```python
from build123d import *

# Parameters (mm, degrees)
SKETCH1_R           = 8
SKETCH1_R_2         = 1.5
SKETCH1_R_3         = 2
SKETCH1_W           = 10
SKETCH1_H           = 10
BOSS_EXTRUDE2_DEPTH = 8


with BuildPart() as part:
    # Sketch1 → Boss-Extrude2 (new body)
    with BuildSketch(Plane.XY):
        with BuildLine():
            Line((18.5, -45), (-18.5, -45))
            ThreePointArc((-18.5, -45), (-21.328427125, -43.828427125), (-22.5, -41))
            Line((-22.5, -41), (-22.5, 41))
            ThreePointArc((-22.5, 41), (-21.328427125, 43.828427125), (-18.5, 45))
            Line((-18.5, 45), (18.5, 45))
            ThreePointArc((18.5, 45), (21.328427125, 43.828427125), (22.5, 41))
            Line((22.5, 41), (22.5, -41))
            ThreePointArc((22.5, -41), (21.328427125, -43.828427125), (18.5, -45))
        make_face()
        Circle(SKETCH1_R, mode=Mode.SUBTRACT)
        with Locations((-11, 0)):
            Circle(SKETCH1_R_2, mode=Mode.SUBTRACT)
        with Locations((-5.5, 9.526279442)):
            Circle(SKETCH1_R_2, mode=Mode.SUBTRACT)
        with Locations((5.5, 9.526279442)):
            Circle(SKETCH1_R_2, mode=Mode.SUBTRACT)
        with Locations((11, 0)):
            Circle(SKETCH1_R_2, mode=Mode.SUBTRACT)
        with Locations((5.5, -9.526279442)):
            Circle(SKETCH1_R_2, mode=Mode.SUBTRACT)
        with Locations((-5.5, -9.526279442)):
            Circle(SKETCH1_R_2, mode=Mode.SUBTRACT)
        with Locations((0, -34.5)):
            Circle(SKETCH1_R_3, mode=Mode.SUBTRACT)
        with Locations((0, 34.5)):
            Circle(SKETCH1_R_3, mode=Mode.SUBTRACT)
        with Locations((-11, -34.5)):
            Rectangle(SKETCH1_W, SKETCH1_H, mode=Mode.SUBTRACT)
        with Locations((11, -34.5)):
            Rectangle(SKETCH1_W, SKETCH1_H, mode=Mode.SUBTRACT)
        with Locations((11, 34.5)):
            Rectangle(SKETCH1_W, SKETCH1_H, mode=Mode.SUBTRACT)
        with Locations((-11, 34.5)):
            Rectangle(SKETCH1_W, SKETCH1_H, mode=Mode.SUBTRACT)
    extrude(amount=BOSS_EXTRUDE2_DEPTH)


solid = part.part
```
Could you check a few things on this model? Use its own coordinates, in mm. A direction names the side the tool comes from. Coordinates: 2 decimals unless noted, no trailing zeros. Write each loop counter-clockwise with the first axis right and the second up, starting at its lowest first coordinate (ties: lowest second). Pieces come first, ordered by that corner, then holes. Notation, with made-up numbers: (5, -39) -> (23, -39) arc R17 cw to (23, -32) -> close; hole circle Ø8 at (-32.75, 52). An arc over 180 degrees is marked (long way). Return JSON: item names as keys, results as strings.
(1) Imagine slicing it at B-B, the plane x = -11. Please give me the cut outline in (y, z).
Numbers:
{"outline": "(-45, 0) -> (-39.5, 0) -> (-39.5, 8) -> (-45, 8) -> close; (-29.5, 0) -> (-1.5, 0) -> (-1.5, 8) -> (-29.5, 8) -> close; (1.5, 0) -> (29.5, 0) -> (29.5, 8) -> (1.5, 8) -> close; (39.5, 0) -> (45, 0) -> (45, 8) -> (39.5, 8) -> close"}
(2) Imagine slicing it at C-C, the plane z = 7. Count the separate pieces of the cut face and the enclosed holes in it, then the cut area to 3 significant figures.
Numbers:
{"separate pieces": "1", "enclosed holes": "13", "area": "3,370 mm2"}
(3) We'd pull the mould along Y, two halves only. Please class faces 3 (the flat face through (0, -45, 4)), 4 (the flat face through (11, 29.5, 4)), 5 (the cylindrical face through (21.297, 43.859, 3.944)), 6 (the flat face through (-22.5, -1, 4)): +Y half, -Y half, draft (parallel to the pull), parting line (faces both ways), or undercut.
Numbers:
{"face 3": "-Y half", "face 4": "undercut", "face 5": "+Y half", "face 6": "draft"}
(4) Which directions (+Z, -Z, +X, -X, +Y, -Y) give clear straight access to the entire face, cutting with the end or side of a thin tool? Please do faces 1 (the flat face through (22.5, 1, 4)), 2 (the flat face through (-11, 39.5, 4)).
Numbers:
{"face 1": "+Z, -Z, +X, +Y, -Y", "face 2": "+Z, -Z"}
(5) Imagine slicing it at A-A, the plane y = 0. Please give me the cut outline in (x, z).
Numbers:
{"outline": "(-22.5, 0) -> (-12.5, 0) -> (-12.5, 8) -> (-22.5, 8) -> close; (-9.5, 0) -> (-8, 0) -> (-8, 8) -> (-9.5, 8) -> close; (8, 0) -> (9.5, 0) -> (9.5, 8) -> (8, 8) -> close; (12.5, 0) -> (22.5, 0) -> (22.5, 8) -> (12.5, 8) -> close"}
(6) I need wall thicknesses on L1, parallel to Y at x = 0, z = 5.75; L2, parallel to Y at x = 8.5, z = 7; L3, parallel to X at y = -30, z = 1.5. Which ranges of each line are inside material? Lowest first, please.
Numbers:
{"L1": "y = -45 to -36.5, -32.5 to -8, 8 to 32.5, 36.5 to 45", "L2": "y = -45 to -39.5, -29.5 to 29.5, 39.5 to 45", "L3": "x = -22.5 to -16, -6 to 6, 16 to 22.5"}
